```python
from build123d import *

# Parameters (mm, degrees)
PAD_DEPTH = 5
FILLET_R  = 1


with BuildPart() as part:
    # Sketch → Pad (new body)
    with BuildSketch(Plane.XY):
        Polygon((-45, -10), (45, -10), (45, 10), (55, 10), (55, 15), (-55, 15), (-55, 10), (-45, 10), align=None)
    extrude(amount=PAD_DEPTH)

    # Fillet
    fillet_edges = [part.edges().sort_by_distance(p)[0] for p in [
        (-45, 0, 5),
        (-45, 0, 0),
        (45, 0, 5),
        (45, 0, 0),
    ]]
    fillet(fillet_edges, radius=FILLET_R)


solid = part.part
```
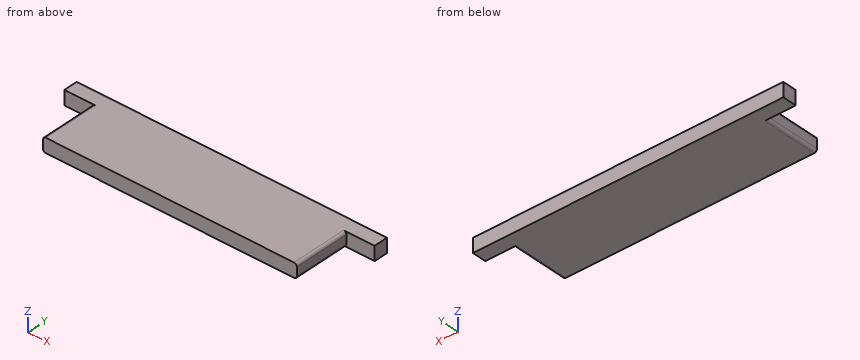
Could you check a few things on this model? Use its own coordinates, in mm. Round coordinates to 2 decimals unless told otherwise and drop trailing zeros. Loops run counter-clockwise (first coordinate to the right, second up) from the corner with the lowest first, then second, coordinate; pieces in that order, holes last. Notation, with made-up numbers: M 36.5,89 L 64.5,89 A25 cw 64.5,108 Z; hole C -1.75,-10 d7. An arc over 180 degrees is marked long. Write item = value, one per line.
1. I need wall thicknesses on probe 1 along X at (y, z) = (8, 2.5); probe 2 along Y at (x, z) = (47, 4.5); probe 3 along X at (y, z) = (-3.75, 4.6). Which ranges of each line are inside material? Lowest first, please.
Results below:
probe_1 = -45 to 45
probe_2 = 10 to 15
probe_3 = -44.8 to 44.8
2. Will these pins go through, and if not, where does the flat tip stop? P1, Ø0.9, axis at y = -0.5, z = 2.5, coming from the +X side; P2, Ø2.5, axis at y = 4.5, z = 3, coming from the -X side; P3, Ø2.5, axis at x = 49, z = 2.5, coming from the -Y side.
Results below:
P1 = 45
P2 = -45
P3 = 10
3. I want a section at B-B, the plane y = 3.5. Write out the boundary of the cut face in (x, z), and give its area (3 significant figures).
Results below:
outline = M -45,1 A1 ccw -44,0 L 44,0 A1 ccw 45,1 L 45,4 A1 ccw 44,5 L -44,5 A1 ccw -45,4 Z
area = 449 mm²
4. I want a section at C-C, the plane x = -47.5. Write out the boundary of the cut face in (y, z), and give its area (3 significant figures).
Results below:
outline = M 10,0 L 15,0 L 15,5 L 10,5 Z
area = 25.0 mm²
5. I want a section at A-A, the plane z = 1.9. Write out the boundary of the cut face in (x, y).
Results below:
outline = M -55,10 L -45,10 L -45,-10 L 45,-10 L 45,10 L 55,10 L 55,15 L -55,15 Z
